```python
from build123d import *

# Parameters (mm, degrees)
SKETCH1_R           = 2
BOSS_EXTRUDE1_DEPTH = 5


with BuildPart() as part:
    # Sketch1 → Boss-Extrude1 (new body)
    with BuildSketch(Plane(origin=(0, 0, 0), x_dir=(1, 0, 0), z_dir=(0, 1, 0))):
        Polygon((-96.706170089, 167.5), (-134.559255134, 101.936533479), (-87.79388333, 74.936533479), (-108.79388333, 38.563466521), (-155.559255134, 65.563466521), (-193.412340179, 0), (-96.706170089, -167.5), (-21, -167.5), (-21, -113.5), (21, -113.5), (21, -167.5), (96.706170089, -167.5), (193.412340179, 0), (155.559255134, 65.563466521), (108.79388333, 38.563466521), (87.79388333, 74.936533479), (134.559255134, 101.936533479), (96.706170089, 167.5), align=None)
        with Locations(Location((-36, -163.5, 0), (0, 0, 270))):
            Circle(SKETCH1_R, mode=Mode.SUBTRACT)
        with Locations(Location((-36, -117.5, 0), (0, 0, 270))):
            Circle(SKETCH1_R, mode=Mode.SUBTRACT)
        with Locations(Location((-123.595153519, 112.926914536, 0), (0, 0, 270))):
            Circle(SKETCH1_R, mode=Mode.SUBTRACT)
        with Locations(Location((-83.757984945, 89.926914536, 0), (0, 0, 270))):
            Circle(SKETCH1_R, mode=Mode.SUBTRACT)
        with Locations(Location((159.595153519, 50.573085464, 0), (0, 0, 270))):
            Circle(SKETCH1_R, mode=Mode.SUBTRACT)
        with Locations(Location((119.757984945, 27.573085464, 0), (0, 0, 270))):
            Circle(SKETCH1_R, mode=Mode.SUBTRACT)
    extrude(amount=BOSS_EXTRUDE1_DEPTH)


solid = part.part
```
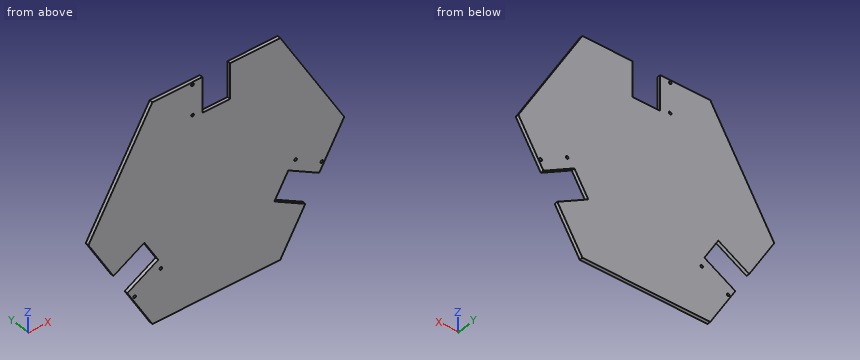
CAD build for the part. Positions are in the model's coordinates, mm. Coordinates: 2 decimals unless noted, no trailing zeros. Loops run counter-clockwise (first coordinate to the right, second up) from the corner with the lowest first, then second, coordinate; pieces in that order, holes last. Notation, with made-up numbers: (-11.75, -22.75) - (4.25, -22.75) arc R24 ccw to (4.25, -4.75) - close; hole circle Ø10 at (-0.75, 77). An arc over 180 degrees is marked (long way). Use CSV: the item, a comma, the result in double quotes. Start each with the question number.
Q1. Cut at D-D, the plane x = -140. List the corners of the cut face in (y, z).
Q2. Drop flat-ended pins along their axis: P1, Ø2.5, axis at x = -36, z = 117.5, coming from the -Y side; P2, Ø2.5, axis at y = 3, z = 140.5, coming from the -X side; P3, Ø5, axis at x = -36, z = 163.5, coming from the -Y side; P4, Ø1.5, axis at y = 3, z = 128.5, coming from the +X side. Give the stop position or say it passes through.
Q3. Probe probe 1 along X at (y, z) = (1.3, -41); probe 2 along X at (y, z) = (3, 117.5); probe 3 along X at (y, z) = (1.1, 114). List the from-to ranges inside material, lowest first. Write a range as from..to.
Q4. Cut at C-C, the plane z = 107. List the corners of the cut face in (x, y).
Q5. Cut at A-A, the plane x = 128. List the corners of the cut face in (y, z).
Q6. Cut at B-B, the plane y = 3.45. List the corners of the cut face in (x, z).
Here are the results:
1,outline,"(0, -56.58) - (5, -56.58) - (5, 92.51) - (0, 92.51) - close"
2,P1,"through"
2,P2,"x = -113.02"
2,P3,"y = 0"
2,P4,"x = 119.66"
3,probe 1,"-169.74..-113.01, -107.39..107.39, 113.01..169.74"
3,probe 2,"-125.57..-38, -34..-21, 21..125.57"
3,probe 3,"-127.59..-21, 21..127.59"
4,outline,"(-131.64, 0) - (131.64, 0) - (131.64, 5) - (-131.64, 5) - close"
5,outline,"(0, -113.3) - (5, -113.3) - (5, -98.15) - (0, -98.15) - close; (0, -49.65) - (5, -49.65) - (5, 113.3) - (0, 113.3) - close"
6,outline,"(-193.41, 0) - (-155.56, -65.56) - (-108.79, -38.56) - (-87.79, -74.94) - (-134.56, -101.94) - (-96.71, -167.5) - (96.71, -167.5) - (134.56, -101.94) - (87.79, -74.94) - (108.79, -38.56) - (155.56, -65.56) - (193.41, 0) - (96.71, 167.5) - (21, 167.5) - (21, 113.5) - (-21, 113.5) - (-21, 167.5) - (-96.71, 167.5) - close; hole circle Ø4 at (-123.6, -112.93); hole circle Ø4 at (-83.76, -89.93); hole circle Ø4 at (-36, 117.5); hole circle Ø4 at (-36, 163.5); hole circle Ø4 at (119.76, -27.57); hole circle Ø4 at (159.6, -50.57)"
